Autodesk Inventor part; units mm, degrees
ref_plane "YZ Plane" through (0, 0, 0) normal (1, 0, 0) x (0, 1, 0)
ref_plane "XZ Plane" through (0, 0, 0) normal (0, 1, 0) x (-1, 0, 0)
ref_plane "XY Plane" through (0, 0, 0) normal (0, 0, 1) x (1, 0, 0)
sketch "Sketch1" plane through (0, 0, 0) normal (0, 0, 1) x (1, 0, 0)
  circle A0 centre (0, 0) radius 6.35
  line L0 (0, 6.35) -> (0, 7.85)
  line L1 (0, 7.85) -> (-1.25, 7.85)
  line L2 (-1.25, 7.85) -> (-1.25, 6.2258)
  line L3 (-5.5508, 5.5508) -> (-6.4347, 4.6669)
  line L4 (-6.4347, 4.6669) -> (-5.2862, 3.5184)
  line L5 (-4.4901, 4.4901) -> (-5.5508, 5.5508)
  line L6 (-7.85, 0) -> (-7.85, -1.25)
  line L7 (-7.85, -1.25) -> (-6.2258, -1.25)
  line L8 (-6.35, 0) -> (-7.85, 0)
  line L9 (-5.5508, -5.5508) -> (-4.6669, -6.4347)
  line L10 (-4.6669, -6.4347) -> (-3.5184, -5.2862)
  line L11 (-4.4901, -4.4901) -> (-5.5508, -5.5508)
  line L12 (0, -7.85) -> (1.25, -7.85)
  line L13 (1.25, -7.85) -> (1.25, -6.2258)
  line L14 (0, -6.35) -> (0, -7.85)
  line L15 (5.5508, -5.5508) -> (6.4347, -4.6669)
  line L16 (6.4347, -4.6669) -> (5.2862, -3.5184)
  line L17 (4.4901, -4.4901) -> (5.5508, -5.5508)
  line L18 (7.85, 0) -> (7.85, 1.25)
  line L19 (7.85, 1.25) -> (6.2258, 1.25)
  line L20 (6.35, 0) -> (7.85, 0)
  line L21 (5.5508, 5.5508) -> (4.6669, 6.4347)
  line L22 (4.6669, 6.4347) -> (3.5184, 5.2862)
  line L23 (4.4901, 4.4901) -> (5.5508, 5.5508)
  circle A1 centre (0, 0) radius 1.625
  point P0 (-3.5184, -5.2862)
  point P1 (4.4901, -4.4901)
  point P2 (5.2862, -3.5184)
  point P3 (6.2258, 1.25)
  point P4 (3.5184, 5.2862)
  dimension "d2" = 1.5
  dimension "d6" = 360
  dimension "d10" = 3.25
extrude "Extrusion1" add sketch "Sketch1" along normal blind 5
properties part number "motor gear"
Build history of the part. All positions in model axes, mm. A direction names the side the tool comes from. Round coordinates to 2 decimals unless told otherwise and drop trailing zeros. Loops run counter-clockwise (first coordinate to the right, second up) from the corner with the lowest first, then second, coordinate; pieces in that order, holes last. Notation, with made-up numbers: (50, 87.25) -> (83, 87.25) arc R25 cw to (83, 104.25) -> close; hole circle Ø2 at (8.5, 54.5). An arc over 180 degrees is marked (long way). Use CSV: the item, a comma, the result in double quotes. Start each with the question number.
Q1. Flat gauge pins, fed straight in: pin 1 Ø1.6 at (x, z) = (-7, 1.5) entering from +Y; pin 2 Ø1.8 at (y, z) = (-7.5, 2.5) entering from +X; pin 3 Ø2 at (x, z) = (-5, 1.5) entering from -Y; pin 4 Ø1 at (y, z) = (-1.5, 3) entering from -X. Where does each tip first touch, or does it go through?
Q2. Saw through at D-D on x = 2.25. Give the cut face in (y, z).
Q3. Saw through at B-B on y = -0.25. Give the cut face in (x, z), and give its area (3 significant figures).
Q4. Which spindle directions (+Z, -Z, +X, -X, +Y, -Y) get a long thin tool onto all of the face, cutting with end or side? Do faces 4 (the face through (-5.585, -3.021, 2.465)), 5 (the face through (5.585, 3.021, 2.465)), 6 (the face through (7, 1.25, 2)), 7 (the face through (1.25, -7, 2)), 8 (the face through (3.021, -5.585, 2.465)). Say none if no direction does.
Q5. Drill centre lines: L1, parallel to Y at x = 7.25, z = 1; L2, parallel to X at y = 2.5, z = 1.75. Where is each one in solid material? Low to high.
Q6. Saw through at C-C on y = 5. Give the cut face in (x, z), and give its area (3 significant figures).
Q7. Mould opens along Y. For faces 1 (the face through (-1.29, 0.99, 2.46)), 2 (the face through (-1.813, -6.086, 2.465)), 3 (the face through (5.1, 6, 2.5)) say: +Y half, -Y half, draft (parallel to the pull), parting line (faces both ways), or undercut.
Solutions:
1,pin 1,"stops at y = 4.9"
1,pin 2,"stops at x = 1.25"
1,pin 3,"stops at y = -6.43"
1,pin 4,"stops at x = -7.85"
2,outline,"(-5.94, 0) -> (5.94, 0) -> (5.94, 5) -> (-5.94, 5) -> close"
3,outline,"(-7.85, 0) -> (-1.61, 0) -> (-1.61, 5) -> (-7.85, 5) -> close; (1.61, 0) -> (6.35, 0) -> (6.35, 5) -> (1.61, 5) -> close"
3,area,"54.9 mm^2"
4,face 4,"+Z, -Z, -X"
4,face 5,"+Z, -Z, +X"
4,face 6,"+Z, -Z, +X, +Y"
4,face 7,"+Z, -Z, +X, -Y"
4,face 8,"+Z, -Z, -Y"
5,L1,"y = 0 to 1.25"
5,L2,"x = -5.84 to 5.84"
6,outline,"(-6.1, 0) -> (-5, 0) -> (-5, 5) -> (-6.1, 5) -> close; (-3.91, 0) -> (5, 0) -> (5, 5) -> (-3.91, 5) -> close"
6,area,"50.1 mm^2"
7,face 1,"undercut"
7,face 2,"-Y half"
7,face 3,"+Y half"
